Here's how the part is built. I have some questions about the finished solid (model axes, mm). A direction names the side the tool comes from. Give positions to 0.01 mm unless a question says otherwise; leave off trailing zeros. Loops run counter-clockwise (first coordinate to the right, second up) from the corner with the lowest first, then second, coordinate; pieces in that order, holes last. Notation, with made-up numbers: (37, 28) - (84, 28) arc R21 ccw to (84, 37) - close; hole circle Ø11 at (5.25, 23). An arc over 180 degrees is marked (long way). Use a Markdown table: item, result.
from build123d import *

# Parameters (mm, degrees)
F1_DEPTH = 9.525
F2_R     = 7.14375
F3_DEPTH = 25.4


with BuildPart() as f1:
    # F0 (on Front) → F1 (new body)
    with BuildSketch(Plane.XZ):
        Polygon((59.556728, 9.525), (48.558205, 9.525), (43.058944, 0), (48.558205, -9.525), (59.556728, -9.525), (65.055989, 0), align=None)
    extrude(amount=F1_DEPTH)

    # F2 (on face) → F3 (join)
    with BuildSketch(Plane(origin=(0, 0, 0), x_dir=(-1, 0, 0), z_dir=(0, 1, 0))):
        with Locations((-54.057466, 0)):
            Circle(F2_R)
    extrude(amount=F3_DEPTH)


solid = f1.part
(1) Will these pins go through, and if not, where does the flat tip stop? pin 1 (6 mm diameter, centred on y = 17.5, z = 2.5, fed in from -X); pin 2 (4 mm diameter, centred on x = 49, y = 13, fed in from +Z); pin 3 (10 mm diameter, centred on y = 2, z = -3, fed in from +X); pin 4 (3 mm diameter, centred on y = 18.5, z = -1.5, fed in from +X).
A:
| item | result |
|---|---|
| pin 1 | x = 46.91 |
| pin 2 | z = 6.46 |
| pin 3 | x = 65.06 |
| pin 4 | x = 61.2 |
(2) Suppose I cut it at C-C on y = 12. Write out the boundary of the cut face in (x, z), plus the area to 3 significant figures.
A:
| item | result |
|---|---|
| outline | circle Ø14.29 at (54.06, 0) |
| area | 160 mm2 |
(3) On a 3-axis mill with a long thin cutter (end or side, diameter ignored), from which of +Z, -Z, +X, -X, +Y, -Y can I reach the whole of each face in a straight line? I mean faces 1 (the face through (61.194, 12.522, 0.314)), 2 (the face through (54, -5, 9.525)). Say none if no direction works.
A:
| item | result |
|---|---|
| face 1 | +Y |
| face 2 | +Z, +X, -X, +Y, -Y |
(4) Suppose I cut it at B-B on x = 52.25. Write out the boundary of the cut face in (y, z) (3 decimals).
A:
| item | result |
|---|---|
| outline | (-9.525, -9.525) - (0, -9.525) - (0, -6.911) - (25.4, -6.911) - (25.4, 6.911) - (0, 6.911) - (0, 9.525) - (-9.525, 9.525) - close |
(5) Suppose I cut it at A-A on z = 5.5. Write out the boundary of the cut face in (x, y) (3 decimals).
A:
| item | result |
|---|---|
| outline | (46.234, -9.525) - (61.881, -9.525) - (61.881, 0) - (58.616, 0) - (58.616, 25.4) - (49.499, 25.4) - (49.499, 0) - (46.234, 0) - close |
(6) If I drill on line 1 (Y direction, x = 61.75, z = -4.25) (3 decimals); line 2 (Z direction, x = 54.25, y = 10.5); line 3 (X direction, y = 10, z = -5.25), over which ranges is the centre line in solid material (lowest first)?
A:
| item | result |
|---|---|
| line 1 | -9.525 to 0 |
| line 2 | -7.14 to 7.14 |
| line 3 | 49.21 to 58.9 |
(7) Suppose I cut it at D-D on x = 45.25. Write out the boundary of the cut face in (y, z) (3 decimals), plus the area to 3 significant figures.
A:
| item | result |
|---|---|
| outline | (-9.525, -3.795) - (0, -3.795) - (0, 3.795) - (-9.525, 3.795) - close |
| area | 72.3 mm2 |
